Work out the finished part from the listing and answer in its coordinate system (mm). Face numbers are marked on the shaded views. A direction names the side the tool comes from. Round coordinates to 2 decimals unless told otherwise and drop trailing zeros. Loops run counter-clockwise (first coordinate to the right, second up) from the corner with the lowest first, then second, coordinate; pieces in that order, holes last. Notation, with made-up numbers: (-27, -17) -> (29, -17) arc R23 cw to (29, 4) -> close; hole circle Ø6 at (49.5, 73). An arc over 180 degrees is marked (long way). Use one line per item in the form item = value.
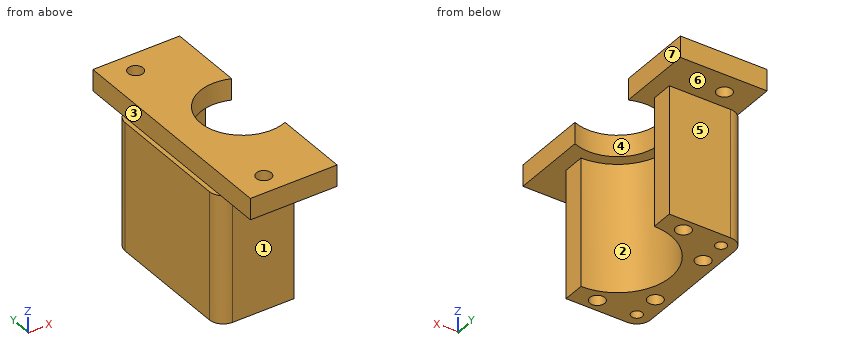
Autodesk Inventor part; units mm, degrees
ref_plane "Work Plane4" through (-37.83, -24.85, 0) normal (0, 0, -1) x (0, 1, 0)
ref_plane "YZ Plane" through (0, 0, 0) normal (1, 0, 0) x (0, 1, 0)
ref_plane "XZ Plane" through (0, 0, 0) normal (0, 1, 0) x (-1, 0, 0)
ref_plane "Work Plane3" through (-9.83, 0, 22) normal (0, 0, -1) x (0, -1, 0)
sketch "Sketch2" plane through (-9.83, 0, 22) normal (0, 0, -1) x (0, -1, 0)
  arc A0 (-15.4, 8) -> (-19.6, 8) centre (-17.5, 8) ccw
  circle A1 centre (17.5, 8) radius 2.1
  circle A2 centre (-17.5, 8) radius 1.4
  circle A3 centre (17.5, 8) radius 1.4
  arc A4 (-11.5, 14) -> (-14, 11.5) centre (-11.5, 11.5) ccw construction
  arc A5 (14, 11.5) -> (11.5, 14) centre (11.5, 11.5) ccw construction
  line L0 (-21.5, 13.2678) -> (21.5, 13.2678)
  line L1 (21.5, 13.2678) -> (21.5, -3)
  line L2 (-21.5, -3) -> (-21.5, 13.2678)
  arc A6 (-2.1271, -1.5804) -> (-2.4402, 1.0334) centre (0, 0) ccw
  arc A7 (7.2826, -3) -> (-7.2826, -3) centre (0, 0) ccw
  line L3 (21.5, -3) -> (7.2826, -3)
  line L4 (-7.2826, -3) -> (-21.5, -3)
  dimension "d26" = 2.8
  dimension "d27" = 2.8
  dimension "d28" = 4
  dimension "d29" = 4
extrude "Extrusion2" add sketch "Sketch2" along normal blind 4 contours A1 | L0 L1 L3 A7 L4 L2
sketch "Sketch3" plane through (-9.83, 0, 18) normal (0, 0, -1) x (-1, 0, 0)
  circle A0 centre (0, 0) radius 12.75
  circle A1 centre (11.5, 11.5) radius 1.025
  circle A2 centre (11.5, -11.5) radius 1.025
  circle A3 centre (-11.5, -11.5) radius 1.025
  circle A4 centre (-11.5, 11.5) radius 1.025
  line L0 (-11.5, -14.1) -> (11.5, -14.1)
  arc A5 (11.5, -14.1) -> (14.1, -11.5) centre (11.5, -11.5) ccw
  line L1 (14.1, -11.5) -> (14.1, 11.5)
  arc A6 (14.1, 11.5) -> (11.5, 14.1) centre (11.5, 11.5) ccw
  line L2 (11.5, 14.1) -> (-11.5, 14.1)
  arc A7 (-11.5, 14.1) -> (-14.1, 11.5) centre (-11.5, 11.5) ccw
  line L3 (-14.1, 11.5) -> (-14.1, -11.5)
  arc A8 (-14.1, -11.5) -> (-11.5, -14.1) centre (-11.5, -11.5) ccw
  line L4 (-11.5, -14.1) -> (11.5, -14.1)
  line L5 (0, -14.1) -> (0, -12.75)
  line L6 (0, 12.75) -> (0, 14.1)
  line L7 (11.5, 14.1) -> (-11.5, 14.1)
  circle A9 centre (0, 0) radius 10
  line L8 (0, -10) -> (0, -12.75)
  line L9 (0, 10) -> (0, 12.75)
  point P0 (-9.83, 0)
  dimension "d11" = 20
ref_plane "Work Plane4" through (-37.83, -24.85, 0) normal (0, 0, -1) x (0, 1, 0)
extrude "Extrusion3" add sketch "Sketch3" along normal blind 24 contours A0 L8 A9 L9 | A0 L6 L2 A6 L1 A5 L0 L5 picked at (11.7268, -0.9457)
sketch "Sketch4" plane through (-9.83, -14.1, -6) normal (0, 0, -1) x (-1, 0, 0)
  circle A0 centre (4.2632, 2.351) radius 1.4
  circle A1 centre (11.5541, 7.5847) radius 1.4
  arc A2 (0, 4.1) -> (0, 24.1) centre (0, 14.1) ccw
  line L0 (10, 14.1) -> (14.0989, 14.1)
  circle A3 centre (4.2632, 25.849) radius 1.4
  circle A4 centre (11.5541, 20.6153) radius 1.4
  point P0 (-9.83, 14.1)
  dimension "d16" = 2.8
  dimension "d17" = 2.8
extrude "Extrusion4" cut sketch "Sketch4" against normal blind 15
properties part number "30_Cube_Z_Focus_MGN_NEMA_Motoradapter_NEMA11_v3"
(1) Find section C-C, the plane z = 9.5. Write down the section's boundary in (x, y) (3 decimals).
Completed:
outline = (-23.93, -11.5) arc R2.6 ccw to (-21.33, -14.1) -> (-9.83, -14.1) -> (-9.83, -10) arc R10 cw to (-9.83, 10) -> (-9.83, 14.1) -> (-21.33, 14.1) arc R2.6 ccw to (-23.93, 11.5) -> close; hole circle Ø2.05 at (-21.33, -11.5); hole circle Ø2.05 at (-21.33, 11.5)
(2) Find section D-D, the plane z = -0.25. Write down the section's boundary in (x, y) (3 decimals), then the cut area to 3 significant figures.
Completed:
outline = (-23.93, -11.5) arc R2.6 ccw to (-21.33, -14.1) -> (-9.83, -14.1) -> (-9.83, -10) arc R10 cw to (-9.83, 10) -> (-9.83, 14.1) -> (-21.33, 14.1) arc R2.6 ccw to (-23.93, 11.5) -> close; hole circle Ø2.8 at (-21.384, -6.515); hole circle Ø2.8 at (-21.384, 6.515); hole circle Ø2.05 at (-21.33, -11.5); hole circle Ø2.05 at (-21.33, 11.5); hole circle Ø2.8 at (-14.093, -11.749); hole circle Ø2.8 at (-14.093, 11.749)
area = 206 mm2
(3) Given P1, Ø4.5, axis at x = -17.83, y = 17.5, coming from the -Z side; P2, Ø0.7, axis at x = -23.5, y = 5, coming from the +Z side; P3, Ø1.5, axis at y = 15.5, z = 4, coming from the +X side; P4, Ø3, axis at x = -21.5, y = -7, coming from the -Z side, each flat-ended and moving along its own axis, determine where each tip first touches the part or whether it passes through.
Completed:
P1 = 18
P2 = 18
P3 = through
P4 = -6
(4) Consider L1, parallel to Y at x = -17.83, z = 19.4; L2, parallel to Y at x = -21.33, z = 6.5 (3 decimals); L3, parallel to X at y = -17.5, z = 20.6. Determine where each line is inside the solid, lowest interval first.
Completed:
L1 = -21.5 to -18.9, -16.1 to 16.1, 18.9 to 21.5
L2 = -14.1 to -12.525, -10.475 to -7.914, -5.116 to 5.116, 7.914 to 10.475, 12.525 to 14.1
L3 = -23.1 to -19.23, -16.43 to -6.83
(5) Find section B-B, the plane x = -9.25. Write down the section's boundary in (y, z), then the cut area to 3 significant figures.
Completed:
outline = (-21.5, 18) -> (-7.85, 18) -> (-7.85, 22) -> (-21.5, 22) -> close; (7.85, 18) -> (21.5, 18) -> (21.5, 22) -> (7.85, 22) -> close
area = 109 mm2
(6) For a pull along Y with two mould halves and no side action, classify the marked faces 4, 5, 6 and 7 as +Y half, -Y half, draft (parallel to the pull), parting line (faces both ways), or undercut.
Completed:
face_4 = undercut
face_5 = +Y half
face_6 = undercut
face_7 = draft
(7) For the marked faces 1, 2 and 3, determine the directions among +Z, -Z, +X, -X, +Y, -Y from which every point of the face is accessible in a straight line to the end or side of a thin tool.
Completed:
face_1 = -Z, +X, -X, -Y
face_2 = -Z, +X
face_3 = +Z, -X, +Y, -Y
(8) Find section A-A, the plane y = -17.5. Write down the section's boundary in (x, z), then the cut area to 3 significant figures.
Completed:
outline = (-23.1, 18) -> (-19.23, 18) -> (-19.23, 22) -> (-23.1, 22) -> close; (-16.43, 18) -> (-6.83, 18) -> (-6.83, 22) -> (-16.43, 22) -> close
area = 53.9 mm2
